Check sheet for the modelled part. Datum: model origin and axes. Units: mm. A direction names the side the tool comes from. Round coordinates to 2 decimals unless told otherwise and drop trailing zeros. Write each loop counter-clockwise with the first axis right and the second up, starting at its lowest first coordinate (ties: lowest second). Pieces come first, ordered by that corner, then holes. Notation, with made-up numbers: (50, 88) -> (106, 88) arc R21 ccw to (106, 107) -> close; hole circle Ø2 at (59.5, 71). An arc over 180 degrees is marked (long way). One line per item, written item: value.
from build123d import *

# Parameters (mm, degrees)
F1_DEPTH = 25.4
F2_R     = 1.5748
F4_DEPTH = 63.5


with BuildPart() as f1:
    # F0 (on Front) → F1 (new body)
    with BuildSketch(Plane.XZ):
        with BuildLine():
            Line((-45.4608029084, -0.1458625454), (32.6695970916, -0.1458625454))
            ThreePointArc((32.6695970916, -0.1458625454), (33.7831488506, 0.3153856956), (34.2443970916, 1.4289374546))
            Line((34.2443970916, 1.4289374546), (34.2443970916, 10.9793374546))
            ThreePointArc((34.2443970916, 10.9793374546), (33.7831488506, 12.0928892136), (32.6695970916, 12.5541374546))
            Line((32.6695970916, 12.5541374546), (-37.1709763854, 12.5541374546))
            ThreePointArc((-37.1709763854, 12.5541374546), (-38.357974904, 13.0940318759), (-38.7310873695, 14.3435271969))
            Line((-38.7310873695, 14.3435271969), (-35.1672138872, 40.2536108012))
            Line((-35.1672138872, 40.2536108012), (-38.9772138872, 40.2536108012))
            Line((-38.9772138872, 40.2536108012), (-47.0356029084, 12.5541374546))
            Line((-47.0356029084, 12.5541374546), (-47.0356029084, 1.4289374546))
            ThreePointArc((-47.0356029084, 1.4289374546), (-46.5743546674, 0.3153856956), (-45.4608029084, -0.1458625454))
        make_face()
    extrude(amount=F1_DEPTH)

    # F2
    f2_edges = [f1.edges().sort_by_distance(p)[0] for p in [
        (-2.25069, -25.4, 12.554137),
        (-2.25069, 0, 12.554137),
        (-35.167214, -12.7, 40.253611),
        (-38.977214, -12.7, 40.253611),
    ]]
    fillet(f2_edges, radius=F2_R)

    # F3 (on face) → F4 (cut)
    with BuildSketch(Plane.YZ.offset(34.2443970916)):
        with BuildLine():
            ThreePointArc((-2.4841372558, 5.9495763853), (-3.6000604195, 8.6436532216), (-6.2941372558, 9.7595763853))
            Line((-6.2941372558, 9.7595763853), (-18.9941372558, 9.7595763853))
            ThreePointArc((-18.9941372558, 9.7595763853), (-21.6882140922, 8.6436532216), (-22.8041372558, 5.9495763853))
            ThreePointArc((-22.8041372558, 5.9495763853), (-21.6882140922, 3.255499549), (-18.9941372558, 2.1395763853))
            Line((-18.9941372558, 2.1395763853), (-6.2941372558, 2.1395763853))
            ThreePointArc((-6.2941372558, 2.1395763853), (-3.6000604195, 3.255499549), (-2.4841372558, 5.9495763853))
        make_face()
    extrude(amount=-F4_DEPTH, mode=Mode.SUBTRACT)


solid = f1.part
Item 1: Sectioned sample at C-C on z = 4. Enter the section's corners in (x, y).
Answer:
outline: (-47.04, -23.83) arc R1.57 ccw to (-45.46, -25.4) -> (32.67, -25.4) arc R1.57 ccw to (34.24, -23.83) -> (34.24, -22.27) -> (-29.26, -22.27) -> (-29.26, -3.02) -> (34.24, -3.02) -> (34.24, -1.57) arc R1.57 ccw to (32.67, 0) -> (-45.46, 0) arc R1.57 ccw to (-47.04, -1.57) -> close
Item 2: Sectioned sample at A-A on x = -9.5. Enter the section's corners in (y, z), and give its area (3 significant figures).
Answer:
outline: (-25.4, 1.43) arc R1.57 ccw to (-23.83, -0.15) -> (-1.57, -0.15) arc R1.57 ccw to (0, 1.43) -> (0, 10.98) arc R1.57 ccw to (-1.57, 12.55) -> (-23.83, 12.55) arc R1.57 ccw to (-25.4, 10.98) -> close; hole (-18.99, 2.14) -> (-6.29, 2.14) arc R3.81 ccw to (-6.29, 9.76) -> (-18.99, 9.76) arc R3.81 ccw to start
area: 178 mm^2
Item 3: Tool access check on faces 1 (the cylindrical face through (-37.39, -24.93, 27.42)), 2 (the flat face through (-43.12, -12.52, 26.02)), 3 (the flat face through (3, -13, 2.14)). Record the directions out of +Z, -Z, +X, -X, +Y, -Y that give a thin tool (end or side, any length) a straight path to the whole face; none if there is none.
Answer:
face 1: +X, -Y
face 2: +Z, -X, +Y, -Y
face 3: +X
Item 4: Depth check by flat-ended pin: P1, Ø6, axis at y = -13, z = 34, coming from the -X side; P2, Ø10, axis at x = -7, y = -15.5, coming from the +Z side; P3, Ø4, axis at y = -12, z = 18, coming from the -X side. Enter the tip coordinate at first touch or a pass-through.
Answer:
P1: stops at x = -41.67
P2: stops at z = 12.55
P3: stops at x = -46.03
Item 5: Thickness scan on line 1 (Z direction, x = -28, y = -12.25); line 2 (X direction, y = -6.5, z = 4.5); line 3 (Y direction, x = -10.5, z = 9). Record the ranges inside material, lowest first.
Answer:
line 1: z = -0.15 to 2.14, 9.76 to 12.55
line 2: x = -47.04 to -29.26
line 3: y = -25.4 to -21.28, -4.01 to 0
Item 6: Sectioned sample at B-B on y = -11. Enter the section's corners in (x, z), and give its area (3 significant figures).
Answer:
outline: (-47.04, 1.43) arc R1.57 ccw to (-45.46, -0.15) -> (32.67, -0.15) arc R1.57 ccw to (34.24, 1.43) -> (34.24, 2.14) -> (-29.26, 2.14) -> (-29.26, 9.76) -> (34.24, 9.76) -> (34.24, 10.98) arc R1.57 ccw to (32.67, 12.55) -> (-37.17, 12.55) arc R1.57 cw to (-38.73, 14.34) -> (-35.41, 38.46) arc R1.57 ccw to (-36.97, 40.25) -> (-37.8, 40.25) arc R1.57 ccw to (-39.31, 39.12) -> (-47.04, 12.55) -> close
area: 711 mm^2
Item 7: Sectioned sample at D-D on y = -20.5. Enter the section's corners in (x, z).
Answer:
outline: (-47.04, 1.43) arc R1.57 ccw to (-45.46, -0.15) -> (32.67, -0.15) arc R1.57 ccw to (34.24, 1.43) -> (34.24, 2.45) -> (-29.26, 2.45) -> (-29.26, 9.45) -> (34.24, 9.45) -> (34.24, 10.98) arc R1.57 ccw to (32.67, 12.55) -> (-37.17, 12.55) arc R1.57 cw to (-38.73, 14.34) -> (-35.41, 38.46) arc R1.57 ccw to (-36.97, 40.25) -> (-37.8, 40.25) arc R1.57 ccw to (-39.31, 39.12) -> (-47.04, 12.55) -> close
Item 8: Mould release check, pull along Z, two halves, no side actions. Record for faces 4 (the cylindrical face through (-5.849, -24.926, 0.303)), 5 (the flat face through (-37.1, -12.5, 26.2)), 6 (the cylindrical face through (-38.729, -12.878, 39.947)): pulls with the +Z half, pulls with the -Z half, needs draft (parallel to the pull), parting line crosses it, or undercut.
Answer:
face 4: pulls with the -Z half
face 5: undercut
face 6: pulls with the +Z half
